Source: CAD feature listing. Evaluate the final solid. Frame: model axes, mm. Give positions to 0.01 mm unless a question says otherwise; leave off trailing zeros. Order: outer loops, then holes, each group sorted by start corner. A loop starts at its lowest first (then second) coordinate and runs counter-clockwise, first axis right, second up. Notation, with made-up numbers: (-35.75, 24.25) - (-17.75, 24.25) arc R26 ccw to (-17.75, 57.25) - close; hole circle Ø2 at (48, 68.5). An arc over 180 degrees is marked (long way). One line per item, written item: value. Start each with the question number.
from build123d import *

# Parameters (mm, degrees)
SKETCH1_W           = 40
SKETCH1_H           = 100
SKETCH1_R           = 2.15
SKETCH1_R_2         = 3.75
BOSS_EXTRUDE2_DEPTH = 3


with BuildPart() as part:
    # Sketch1 → Boss-Extrude2 (new body)
    with BuildSketch(Plane(origin=(0, 0, 0), x_dir=(0, 0, -1), z_dir=(1, 0, 0))):
        with Locations((20, 50)):
            Rectangle(SKETCH1_W, SKETCH1_H)
        with Locations((20, 95)):
            Circle(SKETCH1_R, mode=Mode.SUBTRACT)
        with Locations((20, 5)):
            Circle(SKETCH1_R, mode=Mode.SUBTRACT)
        with Locations((12.5, 50)):
            Circle(SKETCH1_R_2, mode=Mode.SUBTRACT)
        with Locations((27.5, 50)):
            Circle(SKETCH1_R_2, mode=Mode.SUBTRACT)
    extrude(amount=BOSS_EXTRUDE2_DEPTH)


solid = part.part
1. Contact query for flat-ended pins moving along their axis: pin 1 Ø5 at (y, z) = (95, -20) entering from +X; pin 2 Ø6 at (y, z) = (50, -27.5) entering from -X. Output: stop coordinate, or through.
2. Draft query along Z for faces 1 (the flat face through (0, 51, -20)), 2 (the flat face through (1, 49, -40)), 3 (the cylindrical face through (1.48, 46.34, -26.69)), 4 (the flat face through (1, 49, 0)). Return one class per face: pulls with the +Z half, pulls with the -Z half, needs draft (parallel to the pull), parting line crosses it, or undercut.
3. Section C-C on z = -27.5. Return the cut outline in (x, y), then the cut area to 4 significant figures.
4. Section B-B on y = 50. Return the cut outline in (x, z).
5. Section D-D on x = 1.85. Return the cut outline in (y, z).
6. Section A-A on z = -20. Return the cut outline in (x, y).
7. Ray query, L1, parallel to Y at x = 1.2, z = -20; L2, parallel to Y at x = 1.15, z = -27.5; L3, parallel to Y at x = 1.3, z = -9.5. Return the intervals inside material, ascending.
Data:
1. pin 1: stops at x = 3
1. pin 2: passes through
2. face 1: needs draft
2. face 2: pulls with the -Z half
2. face 3: undercut
2. face 4: pulls with the +Z half
3. outline: (0, 0) - (3, 0) - (3, 46.25) - (0, 46.25) - close; (0, 53.75) - (3, 53.75) - (3, 100) - (0, 100) - close
3. area: 277.5 mm2
4. outline: (0, -40) - (3, -40) - (3, -31.25) - (0, -31.25) - close; (0, -23.75) - (3, -23.75) - (3, -16.25) - (0, -16.25) - close; (0, -8.75) - (3, -8.75) - (3, 0) - (0, 0) - close
5. outline: (0, -40) - (100, -40) - (100, 0) - (0, 0) - close; hole circle Ø4.3 at (5, -20); hole circle Ø7.5 at (50, -27.5); hole circle Ø7.5 at (50, -12.5); hole circle Ø4.3 at (95, -20)
6. outline: (0, 0) - (3, 0) - (3, 2.85) - (0, 2.85) - close; (0, 7.15) - (3, 7.15) - (3, 92.85) - (0, 92.85) - close; (0, 97.15) - (3, 97.15) - (3, 100) - (0, 100) - close
7. L1: y = 0 to 2.85, 7.15 to 92.85, 97.15 to 100
7. L2: y = 0 to 46.25, 53.75 to 100
7. L3: y = 0 to 47.75, 52.25 to 100
